```python
from build123d import *

# Parameters (mm, degrees)
F0_W     = 101.6
F0_H     = 88.9
F0_R     = 6.35
F1_DEPTH = 12.7
F2_R     = 2.54
F3_DEPTH = 12.7
F4_W     = 6.35
F4_H     = 82.55
F5_DEPTH = 6.35


with BuildPart() as f1:
    # F0 (on Top) → F1 (new body)
    with BuildSketch(Plane.XY):
        with Locations((-7.979951, 2.434447)):
            Rectangle(F0_W, F0_H)
        Circle(F0_R, mode=Mode.SUBTRACT)
    extrude(amount=-F1_DEPTH)

    # F2
    f2_edges = [f1.edges().sort_by_distance(p)[0] for p in [
        (-58.779951, 2.434447, 0),
        (-7.979951, -42.015553, 0),
        (-7.979951, 46.884447, 0),
        (42.820049, 2.434447, 0),
        (-7.979951, -42.015553, -12.7),
        (-58.779951, -42.015553, -6.35),
        (42.820049, -42.015553, -6.35),
        (42.820049, 2.434447, -12.7),
        (42.820049, 46.884447, -6.35),
        (-7.979951, 46.884447, -12.7),
        (-58.779951, 46.884447, -6.35),
        (-58.779951, 2.434447, -12.7),
    ]]
    fillet(f2_edges, radius=F2_R)

    # F0 (on Top) → F3 (join)
    with BuildSketch(Plane.XY):
        Circle(F0_R)
    extrude(amount=-F3_DEPTH)

    # F4 (on face) → F5 (cut)
    with BuildSketch(Plane.XY):
        with Locations((-41.041727, 1.799447)):
            Rectangle(F4_W, F4_H)
    extrude(amount=-F5_DEPTH, mode=Mode.SUBTRACT)


solid = f1.part
```
The model under review builds one solid part; all positions refer to its coordinate system, in mm. A direction names the side the tool comes from. Round coordinates to 2 decimals unless told otherwise and drop trailing zeros. Order: outer loops, then holes, each group sorted by start corner. A loop starts at its lowest first (then second) coordinate and runs counter-clockwise, first axis right, second up.
(1) Take a section at B-B, the plane y = 9.5. State the section outline as (x, z) points.
Working result:
outline: (-58.78, -10.16) arc R2.54 ccw to (-56.24, -12.7) - (40.28, -12.7) arc R2.54 ccw to (42.82, -10.16) - (42.82, -2.54) arc R2.54 ccw to (40.28, 0) - (-37.87, 0) - (-37.87, -6.35) - (-44.22, -6.35) - (-44.22, 0) - (-56.24, 0) arc R2.54 ccw to (-58.78, -2.54) - close
(2) Mouldability with a two-part tool opening along X and no side actions: class faces 3 (the face through (-37.867, 1, -3)), 4 (the face through (-58.056, 46.121, -6.403)), 5 (the face through (-9, 46.884, -6)) as released by +X, released by -X, zero draft, split by the parting line, or undercut.
Working result:
face 3: undercut
face 4: released by -X
face 5: zero draft
(3) Wall thickness on L1, parallel to X at y = 37.5, z = -5.25; L2, parallel to Y at x = -43.5, z = -3; L3, parallel to X at y = 22.5, z = -10.5: over which ranges is each line inside the solid? List them lowest first.
Working result:
L1: x = -58.78 to -44.22, -37.87 to 42.82
L2: y = -42.02 to -39.48, 43.07 to 46.88
L3: x = -58.76 to 42.8
(4) Tool access review of faces 1 (the face through (-41, 2, -6.35)), 2 (the face through (-7.304, 46.16, -0.764)): name each direction out of +Z, -Z, +X, -X, +Y, -Y from which nothing blocks a thin tool from reaching the whole face with its end or side.
Working result:
face 1: +Z
face 2: +Z, +X, -X, +Y
(5) Take a section at A-A, the plane z = -4. State the section outline as (x, y) points, plus the area to 3 significant figures.
Working result:
outline: (-58.78, -39.48) arc R2.54 ccw to (-56.24, -42.02) - (40.28, -42.02) arc R2.54 ccw to (42.82, -39.48) - (42.82, 44.34) arc R2.54 ccw to (40.28, 46.88) - (-56.24, 46.88) arc R2.54 ccw to (-58.78, 44.34) - close; hole (-44.22, -39.48) - (-37.87, -39.48) - (-37.87, 43.07) - (-44.22, 43.07) - close
area: 8,500 mm2
(6) For P1, Ø1.9, axis at x = -42.5, y = 7.5, coming from the +Z side, flat-tipped, find the tip position at first contact; note if it passes through.
Working result:
P1: stops at z = -6.35
